Here's the drawing with two shaded views (mm, measured from the low corner). I have some questions. A direction names the side the tool comes from. Coordinates: 2 decimals unless noted, no trailing zeros. Loops run counter-clockwise (first coordinate to the right, second up) from the corner with the lowest first, then second, coordinate; pieces in that order, holes last. Notation, with made-up numbers: M 4,-9 L 53,-9 A36 ccw 53,29 Z; hole C 1.25,81.25 d11. An arc over 180 degrees is marked long. Return JSON: item names as keys, results as strings. Group by question number.
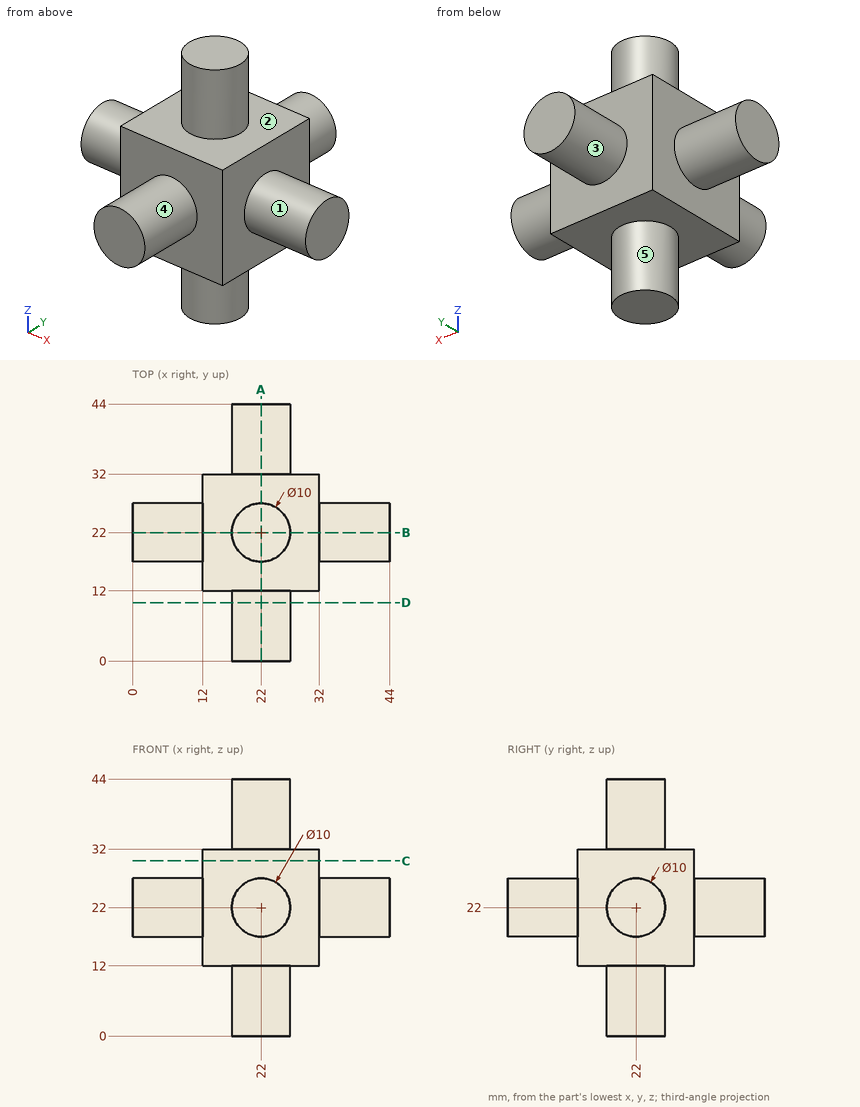
(1) Imagine slicing it at C-C, the plane z = 30. Write out the boundary of the cut face in (x, y), then the cut area to 3 significant figures.
(2) For the marked faces 1, 2, 3, 4 and 5, which set-ups out of +Z, -Z, +X, -X, +Y, -Y let a thin tool reach every point of the face, with its end or its side?
(3) Will these pins go through, and if not, where does the flat tip stop? P1, Ø10, axis at x = 33.5, z = 22.5, coming from the +Y side; P2, Ø1, axis at y = 39, z = 25, coming from the +X side; P3, Ø12, axis at y = 35, z = 33, coming from the -X side.
(4) Imagine slicing it at A-A, the plane x = 22. Write out the boundary of the cut face in (y, z).
(5) If I drill on L1, parallel to X at y = 28, z = 15.5, over which ranges is the centre line in solid material (lowest first)? Write a range as [from, to].
(6) Imagine slicing it at D-D, the plane y = 10. Write out the boundary of the cut face in (x, z).
Checks:
{
 "1": {"outline": "M 12,12 L 32,12 L 32,32 L 12,32 Z", "area": "400 mm²"},
 "2": {"face 1": "+X", "face 2": "+Z", "face 3": "+Y", "face 4": "-Y", "face 5": "-Z"},
 "3": {"P1": "y = 32", "P2": "x = 26.33", "P3": "x = 12"},
 "4": {"outline": "M 0,17 L 12,17 L 12,12 L 17,12 L 17,0 L 27,0 L 27,12 L 32,12 L 32,17 L 44,17 L 44,27 L 32,27 L 32,32 L 27,32 L 27,44 L 17,44 L 17,32 L 12,32 L 12,27 L 0,27 Z"},
 "5": {"L1": "[12, 32]"},
 "6": {"outline": "C 22,22 d10"}
}
